Could you check a few things on this drawing? It's one solid part, dimensions in mm from its lowest x, y, z. A direction names the side the tool comes from. Give positions to 0.01 mm unless a question says otherwise; leave off trailing zeros. Loops run counter-clockwise (first coordinate to the right, second up) from the corner with the lowest first, then second, coordinate; pieces in that order, holes last. Notation, with made-up numbers: (-5.75, -39.75) - (12.25, -39.75) arc R10 cw to (12.25, -32.75) - close; hole circle Ø5 at (70.25, -33.75). An arc over 180 degrees is marked (long way). Write item = value, one per line.
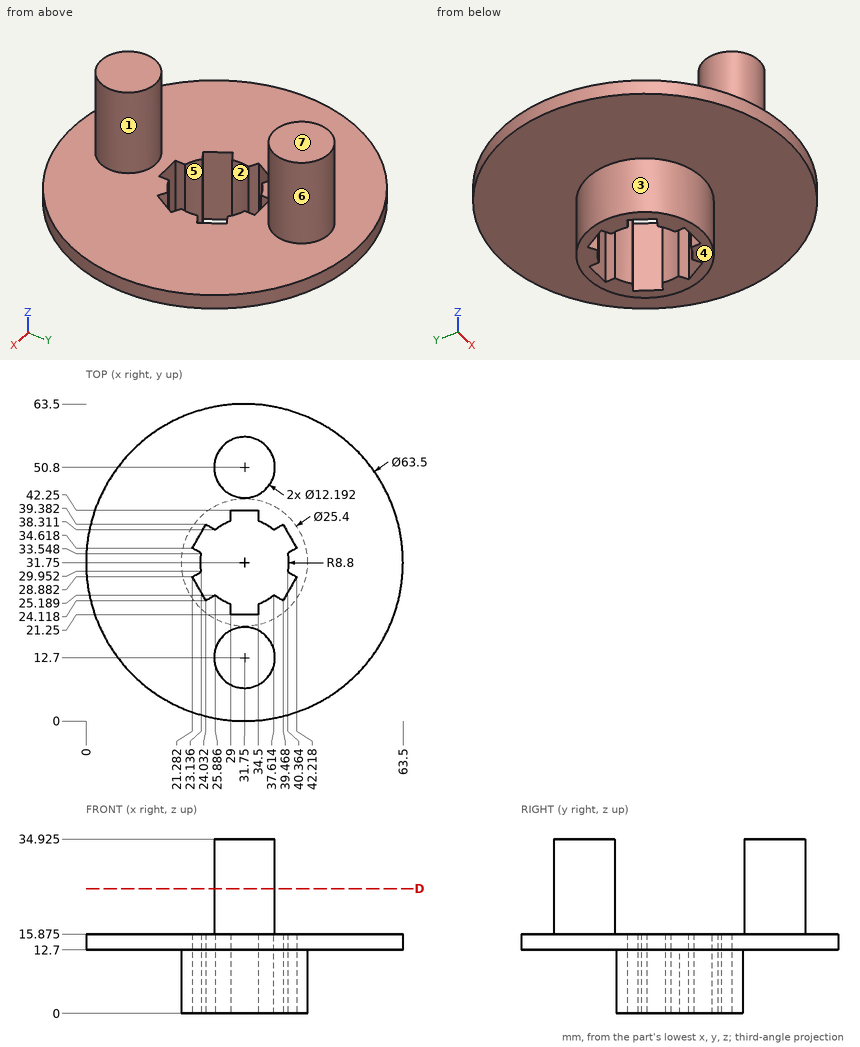
Q1. We'd pull the mould along X, two halves only. Please class the marked faces 5, 6 and 7: released by +X, released by -X, zero draft, split by the parting line, or undercut.
Output:
face_5 = undercut
face_6 = split by the parting line
face_7 = zero draft
Q2. I need wall thicknesses on L1, parallel to Z at x = 57.5, y = 20 (1 decimal); L2, parallel to Y at x = 28, z = 22 (1 decimal); L3, parallel to Z at x = 25, y = 24 (1 decimal). Which ranges of each line are inside material? Lowest first, please.
Output:
L1 = 12.7 to 15.9
L2 = 7.9 to 17.5, 46 to 55.6
L3 = 0 to 15.9
Q3. Imagine slicing it at D-D, the plane z = 25. Write out the boundary of the cut face in (x, y).
Output:
outline = circle Ø12.19 at (31.75, 12.7); circle Ø12.19 at (31.75, 50.8)
Q4. Which directions (+Z, -Z, +X, -X, +Y, -Y) give clear straight access to the entire face, cutting with the end or side of a thin tool? Please do the marked faces 1, 2, 3 and 4.
Output:
face_1 = +Z
face_2 = +Z, -Z
face_3 = -Z
face_4 = -Z, +X, -X, +Y, -Y
Q5. For pin 1 (8 mm diameter, centred on x = 17, z = 16.5, fed in from -Y); pin 2 (6 mm diameter, centred on x = 30.5, z = 6, fed in from +Y); pin 3 (1.6 mm diameter, centred on x = 30.5, z = 10, fed in from -Y), each with a flat end and sliding along its axis, tell me the tip position at first contact or that it passes through.
Output:
pin_1 = 1.89
pin_2 = 44.45
pin_3 = 19.06
